Geometry: final body of the model. Coordinates: model frame, mm. Face numbers are marked on the shaded views. A direction names the side the tool comes from. Round coordinates to 2 decimals unless told otherwise and drop trailing zeros. Order: outer loops, then holes, each group sorted by start corner. A loop starts at its lowest first (then second) coordinate and runs counter-clockwise, first axis right, second up. Notation, with made-up numbers: (36.25, 81) - (43.25, 81) arc R15 ccw to (43.25, 95) - close; hole circle Ø5 at (84, -7.5). An arc over 180 degrees is marked (long way). Put each result on its own line as item: value. Start each with the question number.
(1) Material intervals for L1, parallel to Y at x = 6.5, z = 10.5; L2, parallel to Z at x = 2.75, y = -2.5; L3, parallel to X at y = 0, z = 14, sorted ascending. Write a range as [from, to].
(2) Section D-D (z = 6.5). Output: boundary loops of the cut face in (x, y), and give its area (3 significant figures).
(3) Pull-direction query (Z, two-part tool) for the marked faces 1, 2 and 3; classes: released by +Z, released by -Z, zero draft, split by the parting line, or undercut.
(4) Pin query (flat end, axial travel): P1, Ø1.5, axis at y = 0.5, z = 3.5, coming from the -X side; P2, Ø4, axis at x = 3, z = 13.5, coming from the +Y side; P3, Ø1.5, axis at x = 3, y = 0, coming from the +Z side; P4, Ø2, axis at y = 0, z = 4.5, coming from the +X side. Return the tip coordinate at first contact, or that it passes through.
(5) Section C-C (y = 7). Output: boundary loops of the cut face in (x, z).
(6) Section A-A (x = 0). Output: boundary loops of the cut face in (y, z).
(7) Section B-B (z = 11.75). Output: boundary loops of the cut face in (x, y).
(8) Access query for the marked faces 4, 5 and 6. Directions: +Z, -Z, +X, -X, +Y, -Y. A direction counts if a zero-diameter tool reaches every point of the face in a straight line with its end or side. Return the directions, or none.
Autodesk Fusion 360 part; units mm, degrees
sketch "Sketch1" plane through (0, 0, 0) normal (0, 0, 1) x (1, 0, 0)
  line L0 (9, 9) -> (-9, 9)
  line L1 (-9, 9) -> (-9, -9)
  line L2 (-9, -9) -> (9, -9)
  line L3 (9, -9) -> (9, 9)
  line L4 (9, 9) -> (-9, -9) construction
  line L5 (-9, 9) -> (9, -9) construction
  dimension "d1" = 18
  dimension "d2" = 18
extrude "Extrude1" add sketch "Sketch1" along normal blind 3
sketch "Sketch2" plane through (0, 0, 3) normal (0, 0, 1) x (-1, 0, 0)
  line L0 (-9, 9) -> (-9, -9)
  line L1 (-9, -9) -> (9, -9)
  line L2 (9, -9) -> (9, 9)
  line L3 (9, 9) -> (-9, 9)
  line L4 (2, -1.5) -> (3.5, -1.5)
  line L5 (3.5, -1.5) -> (3.5, 1.5)
  line L6 (3.5, 1.5) -> (2, 1.5)
  line L7 (2, 1.5) -> (2, -1.5)
  line L8 (2, -1.5) -> (3.5, 1.5) construction
  line L9 (3.5, -1.5) -> (2, 1.5) construction
  line L10 (-3.5, -1.5) -> (-2, -1.5)
  line L11 (-2, -1.5) -> (-2, 1.5)
  line L12 (-2, 1.5) -> (-3.5, 1.5)
  line L13 (-3.5, 1.5) -> (-3.5, -1.5)
  line L14 (-3.5, -1.5) -> (-2, 1.5) construction
  line L15 (-2, -1.5) -> (-3.5, 1.5) construction
  line L16 (0, -12) -> (0, 14) construction
  point P0 (2.75, 0)
  point P1 (-2.75, 0)
  dimension "d5" = 3
  dimension "d6" = 1.5
  dimension "d7" = 1.5
  dimension "d8" = 3
  dimension "d9" = 2
extrude "Extrude2" add sketch "Sketch2" along normal blind 2 contours L4 L5 L6 L7 | L10 L11 L12 L13
sketch "Sketch8" plane through (0, 1.5, 0) normal (0, 1, 0) x (-1, 0, 0)
  line L0 (-3.5, 3) -> (-2, 3)
  line L1 (-2, 3) -> (-2, 5)
  line L2 (-2, 5) -> (-3.5, 5)
  line L3 (-3.5, 5) -> (-3.5, 3)
  line L4 (-4.2426, 15.8759) -> (-5.3033, 16.9366)
  line L5 (0, 11.6332) -> (7.5, 11.6332) construction
  line L6 (4.2426, 15.8759) -> (5.3033, 16.9366)
  arc A0 (-5.3033, 16.9366) -> (5.3033, 16.9366) centre (0, 11.6332) ccw
  arc A1 (-4.2426, 15.8759) -> (4.2426, 15.8759) centre (0, 11.6332) ccw
  point P0 (3.5, 5)
  dimension "d18" = 15
  dimension "d19" = 12
  dimension "d20" = 135
extrude "Extrude3" add 1 faces at (-2.5, 1.5, 3.6667) along direction (0, -1, 0) blind 3
extrude "Extrude4" add sketch "Sketch8" against normal blind 3 contours L1 L2 L4 L6 A0 A1
fillet "Fillet1" radius 0.5 2 edges at (-4.2426, 0, 15.8759) (4.2426, 0, 15.8759)
fillet "Fillet2" radius 0.2 4 edges at (9, 0, 0) (0, 9, 0) (-9, 0, 0) (0, -9, 0)
fillet "Fillet3" radius 0.2 2 edges at (5.3033, 0, 16.9366) (-5.3033, 0, 16.9366)
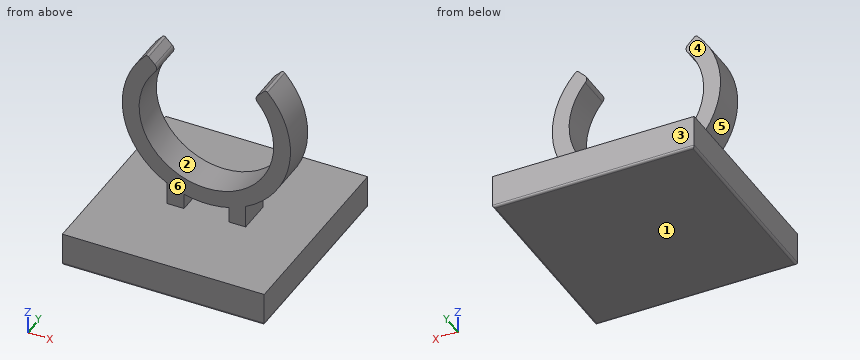
Checks:
1. L1: y = [-1.5, 1.5]
1. L2: z = [0, 3]
1. L3: x = [-7.12, -5.51], [5.51, 7.12]
2. outline: (-5.47, -1.5) - (-3.11, -1.5) - (-3.11, 1.5) - (-5.47, 1.5) - close; (3.11, -1.5) - (5.47, -1.5) - (5.47, 1.5) - (3.11, 1.5) - close
2. area: 14.2 mm²
3. face 1: released by -Z
3. face 2: undercut
3. face 3: zero draft
4. P1: stops at x = -9
4. P2: passes through
4. P3: stops at z = 6.95
4. P4: stops at x = 4.32
5. outline: (-9, 0.2) arc R0.2 ccw to (-8.8, 0) - (8.8, 0) arc R0.2 ccw to (9, 0.2) - (9, 3) - (-9, 3) - close
6. outline: (-9, 0.2) arc R0.2 ccw to (-8.8, 0) - (8.8, 0) arc R0.2 ccw to (9, 0.2) - (9, 3) - (-9, 3) - close; (-1.5, 4.13) - (1.5, 4.13) - (1.5, 5.63) - (-1.5, 5.63) - close
7. outline: (-7.5, -1.5) - (-6, -1.5) - (-6, 1.5) - (-7.5, 1.5) - close; (6, -1.5) - (7.5, -1.5) - (7.5, 1.5) - (6, 1.5) - close
8. face 4: +Z, +X, -X, +Y
8. face 5: -X, +Y, -Y
8. face 6: +Z, +X, -X, -Y
